Geometry check sheet. Reference: the model listing, model coordinates, mm. Round coordinates to 2 decimals unless told otherwise and drop trailing zeros. Order: outer loops, then holes, each group sorted by start corner. A loop starts at its lowest first (then second) coordinate and runs counter-clockwise, first axis right, second up.
(1) Cross-section at B-B on y = 0.85. Count the separate pieces of the cut face and the enclosed holes in it, and give its area (3 significant figures).
(2) Thickness scan on L1, parallel to X at y = 0.4, z = -20; L2, parallel to X at y = 2.5, z = -42.5; L3, parallel to Z at x = 132.5, y = 2.1. Record the ranges inside material, lowest first.
(3) Cross-section at C-C on z = -28. Enter the section's corners in (x, y).
(4) Draft check along X on faces 1 (the face through (143, 3, -35)), 2 (the face through (220.654, 1.479, -40.961)). Enter one of: pulls with the +X half, pulls with the -X half, needs draft (parallel to the pull), parting line crosses it, or undercut.
(5) Gauge pin test, flat end, axial feed: P1, Ø1, axis at y = 1.5, z = -48, coming from the -X side. Record the tip position at first contact, or that the pin passes through.
(6) Cross-section at A-A on x = 177.5. Enter the section's corners in (y, z).
from build123d import *

# Parameters (mm, degrees)
IZIM1_W                     = 290
IZIM1_H                     = 70
IZIM1_R                     = 27.5
IZIM1_R_2                   = 2
Y_KSEKLIK_EKSTR_ZYON1_DEPTH = 3


with BuildPart() as part:
    # Çizim1 → Yükseklik-Ekstrüzyon1 (new body)
    with BuildSketch(Plane(origin=(0, 0, 0), x_dir=(1, 0, 0), z_dir=(0, 1, 0))):
        with Locations((145, 35)):
            Rectangle(IZIM1_W, IZIM1_H)
        with Locations(Location((37.5, 35, 0), (0, 0, 270))):
            Circle(IZIM1_R, mode=Mode.SUBTRACT)
        with Locations(Location((12.5, 60, 0), (0, 0, 270))):
            Circle(IZIM1_R_2, mode=Mode.SUBTRACT)
        with Locations(Location((62.5, 60, 0), (0, 0, 270))):
            Circle(IZIM1_R_2, mode=Mode.SUBTRACT)
        with Locations(Location((62.5, 10, 0), (0, 0, 270))):
            Circle(IZIM1_R_2, mode=Mode.SUBTRACT)
        with Locations(Location((12.5, 10, 0), (0, 0, 270))):
            Circle(IZIM1_R_2, mode=Mode.SUBTRACT)
        with Locations(Location((107.5, 35, 0), (0, 0, 270))):
            Circle(IZIM1_R, mode=Mode.SUBTRACT)
        with Locations(Location((132.5, 60, 0), (0, 0, 270))):
            Circle(IZIM1_R_2, mode=Mode.SUBTRACT)
        with Locations(Location((132.5, 10, 0), (0, 0, 270))):
            Circle(IZIM1_R_2, mode=Mode.SUBTRACT)
        with Locations(Location((82.5, 10, 0), (0, 0, 270))):
            Circle(IZIM1_R_2, mode=Mode.SUBTRACT)
        with Locations(Location((82.5, 60, 0), (0, 0, 270))):
            Circle(IZIM1_R_2, mode=Mode.SUBTRACT)
        with Locations(Location((177.5, 35, 0), (0, 0, 270))):
            Circle(IZIM1_R, mode=Mode.SUBTRACT)
        with Locations(Location((202.5, 60, 0), (0, 0, 270))):
            Circle(IZIM1_R_2, mode=Mode.SUBTRACT)
        with Locations(Location((202.5, 10, 0), (0, 0, 270))):
            Circle(IZIM1_R_2, mode=Mode.SUBTRACT)
        with Locations(Location((152.5, 10, 0), (0, 0, 270))):
            Circle(IZIM1_R_2, mode=Mode.SUBTRACT)
        with Locations(Location((152.5, 60, 0), (0, 0, 270))):
            Circle(IZIM1_R_2, mode=Mode.SUBTRACT)
        with Locations(Location((247.5, 35, 0), (0, 0, 270))):
            Circle(IZIM1_R, mode=Mode.SUBTRACT)
        with Locations(Location((272.5, 60, 0), (0, 0, 270))):
            Circle(IZIM1_R_2, mode=Mode.SUBTRACT)
        with Locations(Location((272.5, 10, 0), (0, 0, 270))):
            Circle(IZIM1_R_2, mode=Mode.SUBTRACT)
        with Locations(Location((222.5, 10, 0), (0, 0, 270))):
            Circle(IZIM1_R_2, mode=Mode.SUBTRACT)
        with Locations(Location((222.5, 60, 0), (0, 0, 270))):
            Circle(IZIM1_R_2, mode=Mode.SUBTRACT)
    extrude(amount=Y_KSEKLIK_EKSTR_ZYON1_DEPTH)


solid = part.part
Found:
1. separate pieces: 1
1. enclosed holes: 20
1. area: 10,600 mm2
2. L1: x = 0 to 14.45, 60.55 to 84.45, 130.55 to 154.45, 200.55 to 224.45, 270.55 to 290
2. L2: x = 0 to 11.04, 63.96 to 81.04, 133.96 to 151.04, 203.96 to 221.04, 273.96 to 290
2. L3: z = -70 to -62, -58 to -46.46, -23.54 to -12, -8 to 0
3. outline: (0, 0) - (10.91, 0) - (10.91, 3) - (0, 3) - close; (64.09, 0) - (80.91, 0) - (80.91, 3) - (64.09, 3) - close; (134.09, 0) - (150.91, 0) - (150.91, 3) - (134.09, 3) - close; (204.09, 0) - (220.91, 0) - (220.91, 3) - (204.09, 3) - close; (274.09, 0) - (290, 0) - (290, 3) - (274.09, 3) - close
4. face 1: needs draft
4. face 2: undercut
5. P1: stops at x = 0
6. outline: (0, -70) - (3, -70) - (3, -62.5) - (0, -62.5) - close; (0, -7.5) - (3, -7.5) - (3, 0) - (0, 0) - close
